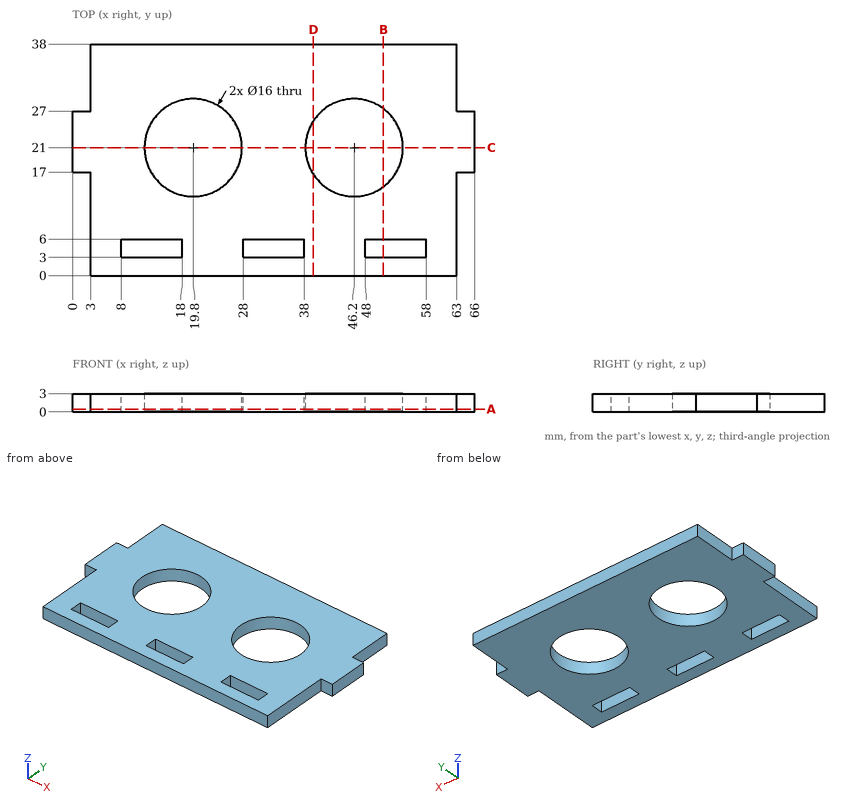
Print and shaded views of the part. All mm, measured from the part's lowest x, y and z. Round coordinates to 2 decimals unless told otherwise and drop trailing zeros. Order: outer loops, then holes, each group sorted by start corner. A loop starts at its lowest first (then second) coordinate and runs counter-clockwise, first axis right, second up.
Q1. Slice it at B-B (x = 51). Write the cut outline in (y, z), and give its area (3 significant figures).
Q2. Slice it at C-C (y = 21). Write the cut outline in (x, z), and give its area (3 significant figures).
Q3. Slice it at D-D (x = 39.5). Write the cut outline in (y, z).
Q4. Drop flat-ended pins along their axis: pin 1 (14.5 mm diameter, centred on x = 46.2, y = 21, fed in from -Z); pin 2 (1.5 mm diameter, centred on y = 30, z = 1.5, fed in from -X); pin 3 (1.5 mm diameter, centred on y = 35, z = 2, fed in from +X); pin 4 (1.5 mm diameter, centred on x = 51, z = 1.5, fed in from -Y). Give the stop position or say it passes through.
Q5. Slice it at A-A (z = 0.45). Write the cut outline in (x, y).
Q6. Wall check: L1, parallel to X at y = 24.5, z = 2.6; L2, parallel to Y at x = 13, z = 1; L3, parallel to X at y = 5.5, z = 2.85. Give the ranges that are in metal, low to high.
Results below:
1. outline: (0, 0) - (3, 0) - (3, 3) - (0, 3) - close; (6, 0) - (14.6, 0) - (14.6, 3) - (6, 3) - close; (27.4, 0) - (38, 0) - (38, 3) - (27.4, 3) - close
1. area: 66.6 mm2
2. outline: (0, 0) - (11.8, 0) - (11.8, 3) - (0, 3) - close; (27.8, 0) - (38.2, 0) - (38.2, 3) - (27.8, 3) - close; (54.2, 0) - (66, 0) - (66, 3) - (54.2, 3) - close
2. area: 102 mm2
3. outline: (0, 0) - (16.63, 0) - (16.63, 3) - (0, 3) - close; (25.37, 0) - (38, 0) - (38, 3) - (25.37, 3) - close
4. pin 1: passes through
4. pin 2: stops at x = 3
4. pin 3: stops at x = 63
4. pin 4: stops at y = 0
5. outline: (0, 17) - (3, 17) - (3, 0) - (63, 0) - (63, 17) - (66, 17) - (66, 27) - (63, 27) - (63, 38) - (3, 38) - (3, 27) - (0, 27) - close; hole (8, 3) - (18, 3) - (18, 6) - (8, 6) - close; hole circle Ø16 at (19.8, 21); hole (28, 3) - (38, 3) - (38, 6) - (28, 6) - close; hole circle Ø16 at (46.2, 21); hole (48, 3) - (58, 3) - (58, 6) - (48, 6) - close
6. L1: x = 0 to 12.61, 26.99 to 39.01, 53.39 to 66
6. L2: y = 0 to 3, 6 to 16.79, 25.21 to 38
6. L3: x = 3 to 8, 18 to 28, 38 to 48, 58 to 63
